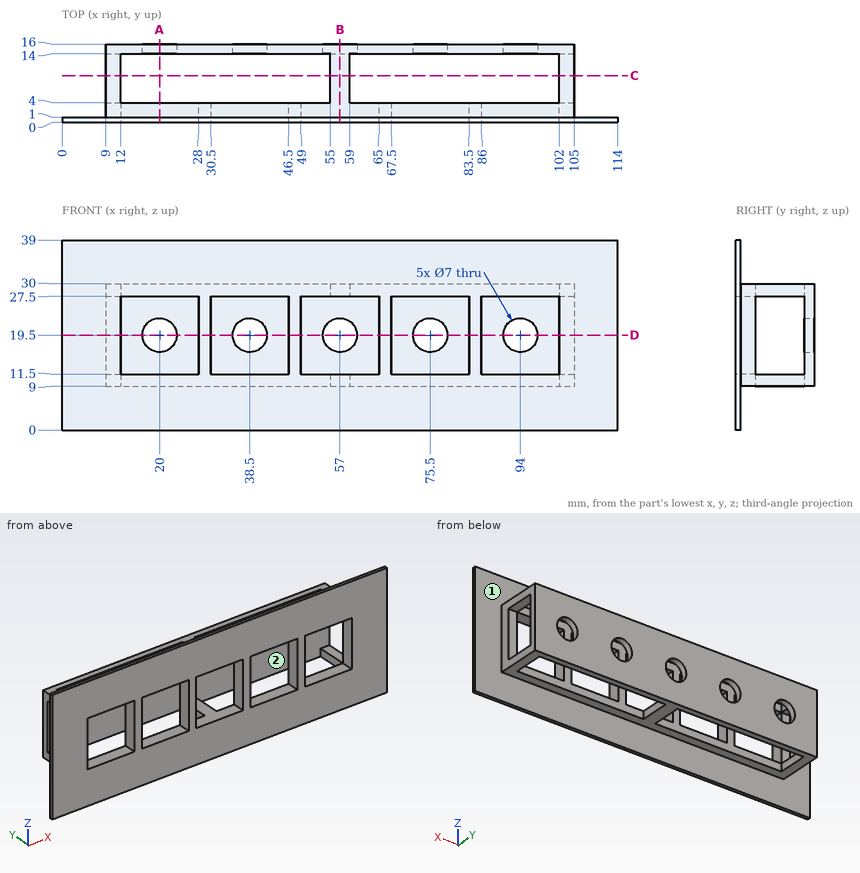
Could you check a few things on this drawing? It's one solid part, dimensions in mm from its lowest x, y, z. Coordinates: 2 decimals unless noted, no trailing zeros. Write each loop counter-clockwise with the first axis right and the second up, starting at its lowest first coordinate (ties: lowest second). Pieces come first, ordered by that corner, then holes.
Q1. Imagine slicing it at B-B, the plane x = 57. List the corners of the cut face in (y, z) for me, plus the area to 3 significant figures.
Results found:
outline: (0, 0) - (1, 0) - (1, 9) - (16, 9) - (16, 16) - (14, 16) - (14, 11.5) - (0, 11.5) - close; (0, 27.5) - (14, 27.5) - (14, 23) - (16, 23) - (16, 30) - (1, 30) - (1, 39) - (0, 39) - close
area: 116 mm2
Q2. If we mould it in two halves opening along X, with no side actions, what happens to the marked faces 1 and 2? For each: +X half, -X half, draft (parallel to the pull), parting line (faces both ways), or undercut.
Results found:
face 1: draft
face 2: undercut
Q3. Imagine slicing it at C-C, the plane y = 9.5. List the corners of the cut face in (x, z) for me, plus the area to 3 significant figures.
Results found:
outline: (9, 9) - (12, 9) - (12, 11.5) - (9, 11.5) - close; (9, 27.5) - (12, 27.5) - (12, 30) - (9, 30) - close; (55, 9) - (59, 9) - (59, 11.5) - (55, 11.5) - close; (55, 27.5) - (59, 27.5) - (59, 30) - (55, 30) - close; (102, 9) - (105, 9) - (105, 11.5) - (102, 11.5) - close; (102, 27.5) - (105, 27.5) - (105, 30) - (102, 30) - close
area: 50.0 mm2
Q4. Imagine slicing it at D-D, the plane z = 19.5. Count the separate pieces of the cut face and the enclosed holes in it, plus the area to 3 significant figures.
Results found:
separate pieces: 12
enclosed holes: 0
area: 204 mm2
Q5. Imagine slicing it at A-A, the plane x = 20. List the corners of the cut face in (y, z) for me.
Results found:
outline: (0, 0) - (1, 0) - (1, 9) - (4, 9) - (4, 11.5) - (0, 11.5) - close; (0, 27.5) - (4, 27.5) - (4, 30) - (1, 30) - (1, 39) - (0, 39) - close; (14, 9) - (16, 9) - (16, 16) - (14, 16) - close; (14, 23) - (16, 23) - (16, 30) - (14, 30) - close
Q6. Please list where these lines run through material, in increasing order: L1, parallel to X at y = 15.3, z = 19.5; L2, parallel to Y at x = 24.5, z = 9.5; L3, parallel to Z at x = 57, y = 15.2.
Results found:
L1: x = 9 to 16.5, 23.5 to 35, 42 to 53.5, 60.5 to 72, 79 to 90.5, 97.5 to 105
L2: y = 0 to 4, 14 to 16
L3: z = 9 to 16, 23 to 30
Q7. For P1, Ø3, axis at y = 2, z = 20.5, coming from the -X side; P2, Ø2, axis at y = 2.5, z = 21, coming from the -X side; P3, Ø1.5, axis at x = 31.5, y = 4, coming from the -Z side; P4, Ø3, axis at x = 64.5, y = 13, coming from the +Z side, each with a flat end and sliding along its axis, tell me the tip position at first contact or that it passes through.
Results found:
P1: stops at x = 0
P2: stops at x = 9
P3: stops at z = 9
P4: stops at z = 30
